from build123d import *

# Parameters (mm, degrees)
SKIZZE1_W                                            = 60
SKIZZE1_H                                            = 30
AUFSATZ_LINEAR_AUSTRAGEN1_DEPTH                      = 70
VERRUNDUNG1_R                                        = 30
STIRNSENKUNG_F_R_M42_ZYLINDERSCHRAUBE_MI_D           = 38
STIRNSENKUNG_F_R_M42_ZYLINDERSCHRAUBE_MI_CBORE_D     = 42
STIRNSENKUNG_F_R_M42_ZYLINDERSCHRAUBE_MI_CBORE_DEPTH = 16
SKIZZE4_R                                            = 22
SCHNITT_LINEAR_AUSTRAGEN1_DEPTH                      = 1
VERRUNDUNG1_OF_SPIEGELN1_R                           = 30
M6_GEWINDEBOHRUNG1_D                                 = 5
M6_GEWINDEBOHRUNG1_DEPTH                             = 20
M6_GEWINDEBOHRUNG1_TIP                               = 1.502151548
VERRUNDUNG2_R                                        = 3


with BuildPart() as part:
    # Skizze1 → Aufsatz-Linear austragen1 (new body)
    with BuildSketch(Plane.XY):
        Rectangle(SKIZZE1_W, SKIZZE1_H)
    aufsatz_linear_austragen1 = extrude(amount=AUFSATZ_LINEAR_AUSTRAGEN1_DEPTH)

    # Verrundung1
    verrundung1_edges = [part.edges().sort_by_distance(p)[0] for p in [
        (30, 0, 70),
        (-30, 0, 70),
    ]]
    fillet(verrundung1_edges, radius=VERRUNDUNG1_R - 0.0001)  # a hair under: the kernel refuses the full size

    # Stirnsenkung für M42 Zylinderschraube mit Innensechskant1 (through all)
    with Locations(Plane(origin=(0, -15, 0), x_dir=(-1, 0, 0), z_dir=(0, -1, 0))):
        with Locations((0, -40)):
            stirnsenkung_f_r_m42_zylinderschraube_mi = CounterBoreHole(STIRNSENKUNG_F_R_M42_ZYLINDERSCHRAUBE_MI_D / 2, STIRNSENKUNG_F_R_M42_ZYLINDERSCHRAUBE_MI_CBORE_D / 2, STIRNSENKUNG_F_R_M42_ZYLINDERSCHRAUBE_MI_CBORE_DEPTH)

    # Skizze4 → Schnitt-Linear austragen1 (cut, symmetric)
    with BuildSketch(Plane(origin=(0, -12, 0), x_dir=(1, 0, 0), z_dir=(0, 1, 0))):
        with Locations(Location((0, -40, 0), (0, 0, 270))):
            Circle(SKIZZE4_R)
    schnitt_linear_austragen1 = extrude(amount=SCHNITT_LINEAR_AUSTRAGEN1_DEPTH, both=True, mode=Mode.SUBTRACT)

    # Spiegeln1: Aufsatz-Linear austragen1, Stirnsenkung für M42 Zylinderschraube mit Innensechskant1, Schnitt-Linear austragen1 across plane
    add(aufsatz_linear_austragen1.mirror(Plane(origin=(30, 15, 70), x_dir=(0, 0, 1), z_dir=(0, -1, 0))))
    add(stirnsenkung_f_r_m42_zylinderschraube_mi.mirror(Plane(origin=(30, 15, 70), x_dir=(0, 0, 1), z_dir=(0, -1, 0))), mode=Mode.SUBTRACT)
    add(schnitt_linear_austragen1.mirror(Plane(origin=(30, 15, 70), x_dir=(0, 0, 1), z_dir=(0, -1, 0))), mode=Mode.SUBTRACT)

    # Verrundung1 of Spiegeln1
    verrundung1_of_spiegeln1_edges = [part.edges().sort_by_distance(p)[0] for p in [
        (30, 30, 70),
        (-30, 30, 70),
    ]]
    fillet(verrundung1_of_spiegeln1_edges, radius=VERRUNDUNG1_OF_SPIEGELN1_R - 0.0001)  # a hair under: the kernel refuses the full size

    # M6 Gewindebohrung1
    with Locations(Plane(origin=(0, 0, 0), x_dir=(-1, 0, 0), z_dir=(0, 0, -1))):
        with Locations((-20, 35), (20, 35), (-20, -5), (20, -5)):
            Hole(M6_GEWINDEBOHRUNG1_D / 2, depth=M6_GEWINDEBOHRUNG1_DEPTH)
            with Locations((0, 0, -(M6_GEWINDEBOHRUNG1_DEPTH + M6_GEWINDEBOHRUNG1_TIP / 2))):  # 118° drill point
                Cone(0, M6_GEWINDEBOHRUNG1_D / 2, M6_GEWINDEBOHRUNG1_TIP, mode=Mode.SUBTRACT)

    # Verrundung2
    verrundung2_edges = [part.edges().sort_by_distance(p)[0] for p in [
        (30, 15, 0),
        (-30, 15, 0),
    ]]
    fillet(verrundung2_edges, radius=VERRUNDUNG2_R)


solid = part.part
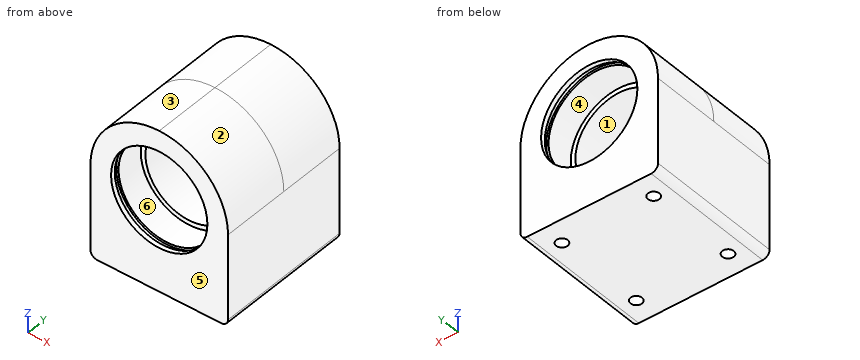
Can you work these out from the model? Positions are in its coordinate system, mm. Face numbers are marked on the shaded views. A direction names the side the tool comes from. Give positions to 0.01 mm unless a question says otherwise; leave off trailing zeros. Answer as a JSON object with one key per item and string values.
Q1. Which directions (+Z, -Z, +X, -X, +Y, -Y) give clear straight access to the entire face, cutting with the end or side of a thin tool? Please do the marked faces 5 and 6.
Geometry says:
{"face 5": "+Z, -Z, +X, -X, -Y", "face 6": "-Y"}
Q2. Will these pins go through, and if not, where does the flat tip stop? P1, Ø12, axis at y = 13, z = 54.5, coming from the +X side; P2, Ø5, axis at x = 8.5, y = 1.5, coming from the +Z side; P3, Ø4, axis at x = -20, y = -5, coming from the +Z side; P4, Ø12.5, axis at x = 10, z = 36, coming from the +Y side.
Geometry says:
{"P1": "x = 28.77", "P2": "z = 69.39", "P3": "z = 64", "P4": "through"}
Q3. If I drill on L1, parallel to X at y = -5, z = 5.25, over which ranges is the centre line in solid material (lowest first)?
Geometry says:
{"L1": "-30 to -22.5, -17.5 to 17.5, 22.5 to 30"}
Q4. If we mould it in two halves opening along X, with no side actions, what happens to the marked faces 1, 2, 3 and 4? For each: pulls with the +X half, pulls with the -X half, needs draft (parallel to the pull), parting line crosses it, or undercut.
Geometry says:
{"face 1": "undercut", "face 2": "pulls with the +X half", "face 3": "pulls with the -X half", "face 4": "undercut"}
